Verification items for this drawing (mm, ordinates from the low corner). Coordinates: 2 decimals unless noted, no trailing zeros. Write each loop counter-clockwise with the first axis right and the second up, starting at its lowest first coordinate (ties: lowest second). Pieces come first, ordered by that corner, then holes. Notation, with made-up numbers: M 13.25,33.25 L 22.25,33.25 A18 cw 22.25,40.25 Z; hole C -13.5,19 d7. An arc over 180 degrees is marked long. Put each result on its own line as item: value. Start each with the question number.
1) Gauge pin test, flat ends, axial feed: pin 1 (8 mm diameter, centred on x = 2, z = 8.5, fed in from +Y); pin 2 (1.5 mm diameter, centred on x = 15.5, z = 27, fed in from -Y). Record the tip position at first contact, or that the pin passes through.
2) Cross-section at B-B on x = 6.25. Record the cut outline in (y, z), plus the area to 3 significant figures.
3) Cross-section at A-A on z = 20. Record the cut outline in (x, y), plus the area to 3 significant figures.
4) Scan lines: line 1 along Y through (x, z) = (10, 21.5); line 2 along X through (y, z) = (1.4, 29). Record each from-to range of solid material in increasing order.
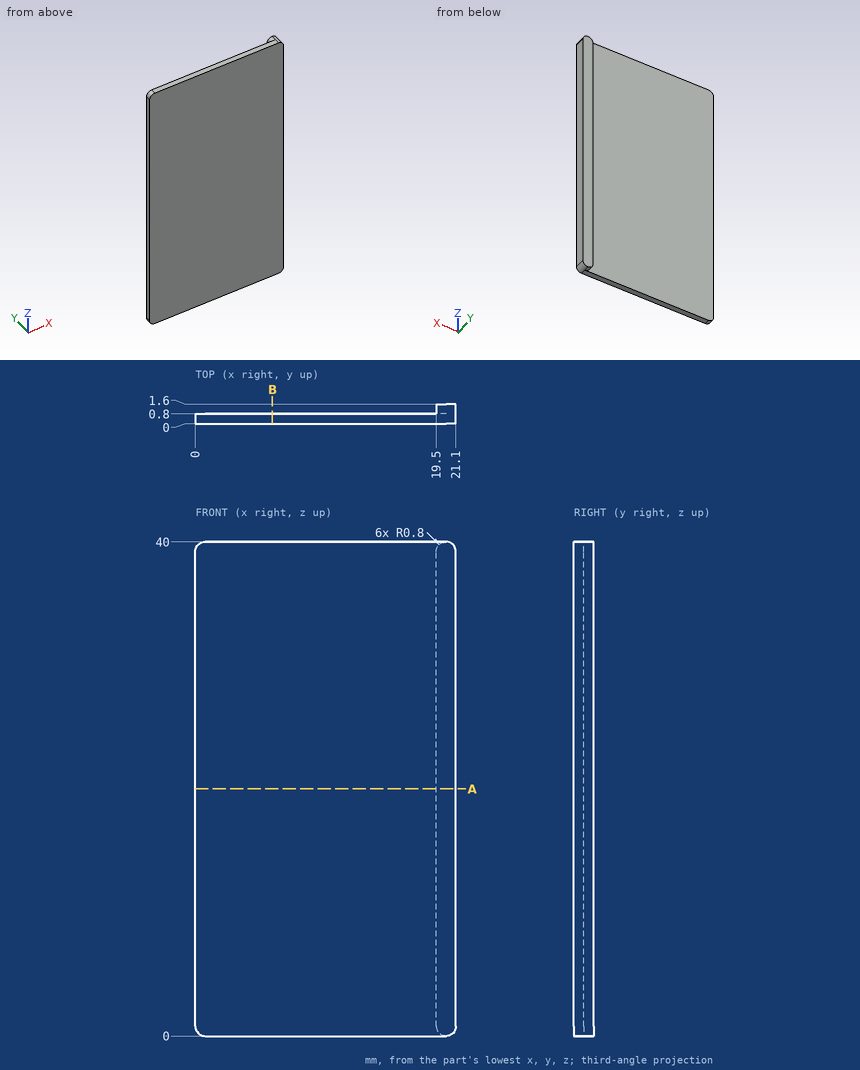
Answer key:
1. pin 1: stops at y = 0.8
1. pin 2: stops at y = 0
2. outline: M 0,0 L 0.8,0 L 0.8,40 L 0,40 Z
2. area: 32.0 mm²
3. outline: M 0,0 L 21.1,0 L 21.1,1.6 L 19.5,1.6 L 19.5,0.8 L 0,0.8 Z
3. area: 18.2 mm²
4. line 1: y = 0 to 0.8
4. line 2: x = 19.5 to 21.1
